```python
from build123d import *

# Parameters (mm, degrees)
BOSS_BASE_DEPTH    = 3
SKETCH3_R          = 2.15
BOSS_FIT_DEPTH     = 2
CUT_SCREWS_START   = -2
SKETCH4_R          = 2.15
CUT_SCREWS_DEPTH   = 2
FILLET1_R          = 2
CUT_VORON_DEPTH    = 0.6
SKETCH8_R          = 9
BOSS_BEARING_DEPTH = 2
SKETCH12_R         = 7.1
CUT_BEARING1_DEPTH = 1.5
SKETCH11_R         = 6
CUT_BEARING2_DEPTH = 157.057681644
CHAMFER2_SIZE      = 3


with BuildPart() as part:
    # Sketch2 → Boss-Base (new body)
    with BuildSketch(Plane.XY):
        with BuildLine():
            Line((-5, 35), (152, 35))
            Line((152, 35), (152, 5))
            ThreePointArc((152, 5), (149.071067812, -2.071067812), (142, -5))
            Line((142, -5), (5, -5))
            ThreePointArc((5, -5), (-2.071067812, -2.071067812), (-5, 5))
            Line((-5, 5), (-5, 35))
        make_face()
    extrude(amount=BOSS_BASE_DEPTH)

    # Sketch3 → Boss-Fit (add)
    with BuildSketch(Plane.XY.offset(3)):
        with BuildLine():
            Line((1, 5), (1, 34.5))
            Line((1, 34.5), (146, 34.5))
            Line((146, 34.5), (146, 5))
            ThreePointArc((146, 5), (144.828427125, 2.171572875), (142, 1))
            Line((142, 1), (5, 1))
            ThreePointArc((5, 1), (2.171572875, 2.171572875), (1, 5))
        make_face()
        with Locations((4.4, 20)):
            Circle(SKETCH3_R, mode=Mode.SUBTRACT)
        with Locations(Location((142.6, 20, 0), (0, 0, 180))):
            Circle(SKETCH3_R, mode=Mode.SUBTRACT)
        with BuildLine():
            Line((2, 33.5), (145, 33.5))
            Line((145, 33.5), (145, 22.547547841))
            ThreePointArc((145, 22.547547841), (139.1, 20), (145, 17.452452159))
            Line((145, 17.452452159), (145, 5))
            ThreePointArc((145, 5), (144.121320344, 2.878679656), (142, 2))
            Line((142, 2), (5, 2))
            ThreePointArc((5, 2), (2.878679656, 2.878679656), (2, 5))
            Line((2, 5), (2, 17.452452159))
            ThreePointArc((2, 17.452452159), (7.9, 20), (2, 22.547547841))
            Line((2, 22.547547841), (2, 33.5))
        make_face(mode=Mode.SUBTRACT)
    extrude(amount=BOSS_FIT_DEPTH)

    # Sketch4 → Cut-Screws (cut)
    with BuildSketch(Plane.XY.offset(3).offset(CUT_SCREWS_START)):
        with Locations((4.4, 20)):
            Circle(SKETCH4_R)
        with Locations(Location((142.6, 20, 0), (0, 0, 180))):
            Circle(SKETCH4_R)
    extrude(amount=CUT_SCREWS_DEPTH, mode=Mode.SUBTRACT)

    # Fillet1
    fillet1_edges = [part.edges().sort_by_distance(p)[0] for p in [
        (152, 20, 0),
        (149.071067812, -2.071067812, 0),
        (73.5, -5, 0),
        (-2.071067812, -2.071067812, 0),
        (-5, 20, 0),
    ]]
    fillet(fillet1_edges, radius=FILLET1_R)

    # Sketch10 → Cut-Voron (cut)
    with BuildSketch(Plane(origin=(0, 0, 0), x_dir=(-1, 0, 0), z_dir=(0, 0, -1))):
        Polygon((-140.798754771, 14), (-145, 8), (-142.25, 8), (-138.048754771, 14), align=None)
        Polygon((-136.048754771, 14), (-144.451245229, 2), (-141.701245229, 2), (-133.298754771, 14), align=None)
        Polygon((-135.5, 8), (-139.701245229, 2), (-136.951245229, 2), (-132.75, 8), align=None)
    extrude(amount=-CUT_VORON_DEPTH, mode=Mode.SUBTRACT)

    # Sketch8 → Boss-Bearing (add)
    with BuildSketch(Plane.XY.offset(3)):
        with Locations((73.5, 24)):
            Circle(SKETCH8_R)
    extrude(amount=BOSS_BEARING_DEPTH)

    # Sketch12 → Cut-Bearing1 (cut)
    with BuildSketch(Plane.XY.offset(5)):
        with Locations((73.5, 24)):
            Circle(SKETCH12_R)
    extrude(amount=-CUT_BEARING1_DEPTH, mode=Mode.SUBTRACT)

    # Sketch11 → Cut-Bearing2 (cut, through all)
    with BuildSketch(Plane.XY.offset(5)):
        with Locations((73.5, 24)):
            Circle(SKETCH11_R)
    extrude(amount=-CUT_BEARING2_DEPTH, mode=Mode.SUBTRACT)

    # Chamfer2
    chamfer2_edges = [part.edges().sort_by_distance(p)[0] for p in [
        (67.5, 24, 0),
    ]]
    chamfer(chamfer2_edges, length=CHAMFER2_SIZE)


solid = part.part
```
Work out the finished part from the listing and answer in its coordinate system (mm). A direction names the side the tool comes from. Round coordinates to 2 decimals unless told otherwise and drop trailing zeros. Order: outer loops, then holes, each group sorted by start corner. A loop starts at its lowest first (then second) coordinate and runs counter-clockwise, first axis right, second up.
Q1. A cutting plane is placed at A-A, the plane x = 73.5. Determine the outline of the cut face in (y, z).
Solution:
outline: (-5, 2) arc R2 ccw to (-3, 0) - (15, 0) - (18, 3) - (18, 3.5) - (16.9, 3.5) - (16.9, 5) - (15, 5) - (15, 3) - (2, 3) - (2, 5) - (1, 5) - (1, 3) - (-5, 3) - close; (30, 3) - (33, 0) - (35, 0) - (35, 3) - (34.5, 3) - (34.5, 5) - (33.5, 5) - (33.5, 3) - (33, 3) - (33, 5) - (31.1, 5) - (31.1, 3.5) - (30, 3.5) - close
Q2. A tool of negligible diameter and unlimited length cuts with its end or side. For faces 1 (the flat face through (140.191, 8.084, 0.296)), 2 (the flat face through (72, 35, 1)), 3 (the cylindrical face through (140.614, 20.823, 2.972)), 4 (the cylindrical face through (144.859, 2.203, 3.986)), from which of +Z, -Z, +X, -X, +Y, -Y can it reach the whole face along a straight path? Write none if from no direction.
Solution:
face 1: -Z
face 2: +Z, -Z, +X, -X, +Y
face 3: +Z
face 4: +Z, +X, -Y
Q3. Given pin 1 Ø1.6 at (y, z) = (17.5, 4) entering from -X; pin 2 Ø1.6 at (x, z) = (72.5, 4.5) entering from -Y; pin 3 Ø0.5 at (x, z) = (135, 0.5) entering from -Y, each flat-ended and moving along its own axis, determine where each tip first touches the part or whether it passes through.
Solution:
pin 1: stops at x = 1
pin 2: stops at y = 1
pin 3: stops at y = -4.56
Q4. A cutting plane is placed at B-B, the plane x = 103.5. Determine the outline of the cut face in (y, z), then the cut area to 3 significant figures.
Solution:
outline: (-5, 2) arc R2 ccw to (-3, 0) - (35, 0) - (35, 3) - (34.5, 3) - (34.5, 5) - (33.5, 5) - (33.5, 3) - (2, 3) - (2, 5) - (1, 5) - (1, 3) - (-5, 3) - close
area: 123 mm2
Q5. Find the intervals of material crossed by line 1 along Y through (x, z) = (73.5, 4.65); line 2 along Y through (x, z) = (17.5, 3.9); line 3 along X through (y, z) = (5, 4), in increasing order.
Solution:
line 1: y = 1 to 2, 15 to 16.9, 31.1 to 33, 33.5 to 34.5
line 2: y = 1 to 2, 33.5 to 34.5
line 3: x = 1 to 2, 145 to 146
